Could you check a few things on this model? Use its own coordinates, in mm. A direction names the side the tool comes from. Coordinates: 2 decimals unless noted, no trailing zeros. Loops run counter-clockwise (first coordinate to the right, second up) from the corner with the lowest first, then second, coordinate; pieces in that order, holes last. Notation, with made-up numbers: (16, 63) - (25, 63) arc R9 cw to (25, 74) - close; hole circle Ø3 at (24.25, 76). An arc over 180 degrees is marked (long way). Put each result on its own line as item: value. Start each with the question number.
```python
from build123d import *

# Parameters (mm, degrees)
SKETCH1_W           = 112
SKETCH1_H           = 125
BOSS_EXTRUDE1_DEPTH = 55
SKETCH2_W           = 110.4
SKETCH2_H           = 123.4
CUT_EXTRUDE1_DEPTH  = 54.2
SKETCH3_W           = 44
SKETCH3_H           = 22
BOSS_EXTRUDE2_DEPTH = 5
SKETCH4_W           = 2.65
SKETCH4_H           = 15
CUT_EXTRUDE2_DEPTH  = 4
SKETCH6_W           = 2.65
SKETCH6_H           = 15
CUT_EXTRUDE3_DEPTH  = 4
FILLET1_R           = 15
FILLET2_R           = 15


with BuildPart() as part:
    # Sketch1 → Boss-Extrude1 (new body)
    with BuildSketch(Plane(origin=(0, 0, 0), x_dir=(1, 0, 0), z_dir=(0, 1, 0))):
        Rectangle(SKETCH1_W, SKETCH1_H)
    extrude(amount=BOSS_EXTRUDE1_DEPTH)

    # Sketch2 → Cut-Extrude1 (cut)
    with BuildSketch(Plane(origin=(0, 55, 0), x_dir=(1, 0, 0), z_dir=(0, 1, 0))):
        Rectangle(SKETCH2_W, SKETCH2_H)
    extrude(amount=-CUT_EXTRUDE1_DEPTH, mode=Mode.SUBTRACT)

    # Sketch3 → Boss-Extrude2 (add)
    with BuildSketch(Plane(origin=(56, 0, 0), x_dir=(0, 0, -1), z_dir=(1, 0, 0))):
        with Locations((-17, 44)):
            Rectangle(SKETCH3_W, SKETCH3_H)
    boss_extrude2 = extrude(amount=BOSS_EXTRUDE2_DEPTH)

    # Sketch4 → Cut-Extrude2 (cut)
    with BuildSketch(Plane.XY.offset(39)):
        with Locations((57.325, 40.5)):
            Rectangle(SKETCH4_W, SKETCH4_H)
    cut_extrude2 = extrude(amount=-CUT_EXTRUDE2_DEPTH, mode=Mode.SUBTRACT)

    # Sketch6 → Cut-Extrude3 (cut)
    with BuildSketch(Plane(origin=(0, 0, -5), x_dir=(-1, 0, 0), z_dir=(0, 0, -1))):
        with Locations((-57.325, 40.5)):
            Rectangle(SKETCH6_W, SKETCH6_H)
    cut_extrude3 = extrude(amount=-CUT_EXTRUDE3_DEPTH, mode=Mode.SUBTRACT)

    # Mirror5: Boss-Extrude2 across plane
    add(boss_extrude2.mirror(Plane(origin=(0, 0, 0), x_dir=(0, 0, 1), z_dir=(1, 0, 0))))

    # Mirror6: Cut-Extrude2 across plane
    add(cut_extrude2.mirror(Plane(origin=(0, 0, 0), x_dir=(0, 0, 1), z_dir=(1, 0, 0))), mode=Mode.SUBTRACT)

    # Mirror7: Cut-Extrude3 across plane
    add(cut_extrude3.mirror(Plane(origin=(0, 0, 0), x_dir=(0, 0, 1), z_dir=(1, 0, 0))), mode=Mode.SUBTRACT)

    # Fillet1
    # the kernel refuses this fillet: 15 mm, written as the material it takes off along each edge
    with BuildSketch(Plane(origin=(61, 33, -32.950849719), x_dir=(-1, 0, 0), z_dir=(0, 0, 1))) as fillet1_piece_1:
        with BuildLine():
            CenterArc((15, -11.180339887), FILLET1_R, 131.810314896, 48.189685104)
            Line((0, -11.180339887), (-0.3, -11.180339887))
            Line((-0.3, -11.180339887), (-0.3, 0))
            Line((-0.3, 0), (0, 0.3))
            ThreePointArc((0, 0.3), (2.5, 0.3), (4.8, 0.223606798))
            Line((4.8, 0.223606798), (5, 0))
        make_face()
    extrude(amount=99.901699437, mode=Mode.SUBTRACT)

    # Fillet2
    # the kernel refuses this fillet: 15 mm, written as the material it takes off along each edge
    with BuildSketch(Plane(origin=(-61, 33, -32.950849719), x_dir=(1, 0, 0), z_dir=(0, 0, 1))) as fillet2_piece_1:
        with BuildLine():
            CenterArc((15, 11.180339887), FILLET2_R, 180, 48.189685104)
            Line((0, 11.180339887), (-0.3, 11.180339887))
            Line((-0.3, 11.180339887), (-0.3, 0))
            Line((-0.3, 0), (0, -0.3))
            ThreePointArc((0, -0.3), (2.5, -0.3), (4.8, -0.223606798))
            Line((4.8, -0.223606798), (5, 0))
        make_face()
    extrude(amount=99.901699437, mode=Mode.SUBTRACT)


solid = part.part
```
(1) I want a section at B-B on x = 8. List the corners of the cut face in (y, z) for me.
(2) I want a section at C-C on z = -48. List the corners of the cut face in (x, y) for me, and give its area (3 significant figures).
(3) I need wall thicknesses on L1, parallel to Z at x = 51.5, y = 5.5; L2, parallel to X at y = 13.5, z = 41; L3, parallel to X at y = 48.5, z = 11.5. Which ranges of each line are inside material? Lowest first, please. Write a range as [from, to].
(4) I want a section at A-A on y = 23. List the corners of the cut face in (x, z) for me.
(5) If we mould it in two halves opening along Z, with no side actions, what happens to faces 5 (the flat face through (59, 48, -5)), 6 (the flat face through (55.2, 28, 1)), 7 (the cylindrical face through (59.66, 37.98, 16.69))? For each: pulls with the +Z half, pulls with the -Z half, needs draft (parallel to the pull), parting line crosses it, or undercut.
(6) Which directions (+Z, -Z, +X, -X, +Y, -Y) give clear straight access to the entire face, cutting with the end or side of a thin tool? Please do faces 1 (the flat face through (-55.2, 28, 1)), 2 (the flat face through (-59, 48, -5)), 3 (the flat face through (-58.65, 42, 37)), 4 (the flat face through (58.65, 42, -3)).
(7) I want a section at D-D on y = 40.5. List the corners of the cut face in (x, z) for me.
(8) For pin 1 Ø2 at (x, z) = (-10, 18) entering from +Y; pin 2 Ø5 at (y, z) = (41.5, -18) entering from -X; pin 3 Ø2 at (y, z) = (42, -3) entering from -X; pin 4 Ø2 at (x, z) = (-26, -18) entering from -Y, each with a flat end and sliding along its axis, tell me the tip position at first contact or that it passes through.
Answer sheet:
1. outline: (0, -62.5) - (55, -62.5) - (55, -61.7) - (0.8, -61.7) - (0.8, 61.7) - (55, 61.7) - (55, 62.5) - (0, 62.5) - close
2. outline: (-56, 0) - (56, 0) - (56, 55) - (55.2, 55) - (55.2, 0.8) - (-55.2, 0.8) - (-55.2, 55) - (-56, 55) - close
2. area: 176 mm^2
3. L1: z = [-62.5, -61.7], [61.7, 62.5]
3. L2: x = [-56, -55.2], [55.2, 56]
3. L3: x = [-61, -55.2], [55.2, 61]
4. outline: (-56, -62.5) - (56, -62.5) - (56, 62.5) - (-56, 62.5) - close; hole (-55.2, -61.7) - (55.2, -61.7) - (55.2, 61.7) - (-55.2, 61.7) - close
5. face 5: pulls with the -Z half
5. face 6: undercut
5. face 7: needs draft
6. face 1: +Y
6. face 2: -Z, -X, +Y, -Y
6. face 3: +Z, -Y
6. face 4: -Z, -Y
7. outline: (-60.54, -5) - (-58.65, -5) - (-58.65, -1) - (-56, -1) - (-56, -62.5) - (56, -62.5) - (56, -1) - (58.65, -1) - (58.65, -5) - (60.54, -5) - (60.54, 39) - (58.65, 39) - (58.65, 35) - (56, 35) - (56, 62.5) - (-56, 62.5) - (-56, 35) - (-58.65, 35) - (-58.65, 39) - (-60.54, 39) - close; hole (-55.2, -61.7) - (55.2, -61.7) - (55.2, 61.7) - (-55.2, 61.7) - close
8. pin 1: stops at y = 0.8
8. pin 2: stops at x = -56
8. pin 3: stops at x = -60.95
8. pin 4: stops at y = 0
